Model file for the job. Use its own axes, mm. A direction names the side the tool comes from. Round coordinates to 2 decimals unless told otherwise and drop trailing zeros. Order: outer loops, then holes, each group sorted by start corner. A loop starts at its lowest first (then second) coordinate and runs counter-clockwise, first axis right, second up. Notation, with made-up numbers: M -33,76.5 L 14,76.5 A6 ccw 14,82.5 Z; hole C -9.75,-21.75 d6. An arc over 180 degrees is marked long. Return JSON: item names as keys, results as strings. Group by question number.
Item 1: Slice it at A-A on x = 105. Write the cut outline in (y, z), then the cut area to 3 significant figures.
Item 2: Which spindle directions (+Z, -Z, +X, -X, +Y, -Y) get a long thin tool onto all of the face, cutting with end or side? Do faces 5 (the face through (162, 117.5, 7)), 6 (the face through (180.505, 12.72, 198.768)), 7 (the face through (161.923, 28.755, 1.232)), 8 (the face through (14.479, 1.232, 188.966)). Say none if no direction does.
Item 3: Slice it at C-C on x = 15. Write the cut outline in (y, z), then the cut area to 3 significant figures.
Item 4: Slice it at B-B on y = 96. Write the cut outline in (x, z), then the cut area to 4 significant figures.
Item 5: Pin check, flat tips, straight feed: pin 1 Ø5 at (x, z) = (250.5, 37.5) entering from +Y; pin 2 Ø3 at (x, y) = (277.5, 115) entering from -Z. Stop position of each tip, or through.
Item 6: Probe line 1 along X through (y, z) = (25, 0.85); line 2 along Y through (x, z) = (195, 1.6); line 3 along X through (y, z) = (12, 145.5). List the from-to ranges inside material, lowest first.
Item 7: Slice it at D-D on z = 34. Write the cut outline in (x, y), then the cut area to 3 significant figures.
Item 8: Pull direction Y, two halves, no side cores. Call faces 1 (the face through (149, 120, 188)), 2 (the face through (148, 61, 0)), 3 (the face through (148.505, 12.72, 198.768)), 4 (the face through (148, 0, 99)): pulls with the +Y half, pulls with the -Y half, needs draft (parallel to the pull), parting line crosses it, or undercut.
from build123d import *

# Parameters (mm, degrees)
F0_W      = 300
F0_H      = 120
F1_DEPTH  = 200
F2_T      = -2.5
F3_W      = 297.5
F3_H      = 197.5
F3_W_2    = 277.5
F3_H_2    = 177.5
F4_DEPTH  = 2.5
F5_R      = 2
F6_DEPTH  = 200.001
F7_R      = 5
F8_DEPTH  = 5
F9_R      = 4
F10_DEPTH = 2.5
F11_R     = 12.5
F12_DEPTH = 3


with BuildPart() as f1:
    # F0 (on Top) → F1 (new body)
    with BuildSketch(Plane.XY):
        with Locations((150, 60)):
            Rectangle(F0_W, F0_H)
    extrude(amount=F1_DEPTH)

    # F2
    f2_openings = [f1.faces().sort_by_distance(p)[0] for p in [
        (150, 120, 100),
    ]]
    offset(amount=F2_T, openings=f2_openings)

    # F3 (on face) → F4 (join)
    with BuildSketch(Plane(origin=(0, 120, 0), x_dir=(-1, 0, 0), z_dir=(0, 1, 0))):
        with Locations((-148.75, 98.75)):
            Rectangle(F3_W, F3_H)
        with Locations((-148.75, 98.75)):
            Rectangle(F3_W_2, F3_H_2, mode=Mode.SUBTRACT)
    extrude(amount=-F4_DEPTH)

    # F5 (on face) → F6 (cut, through all)
    with BuildSketch(Plane.XY.offset(200)):
        with Locations((277.5, 115)):
            Circle(F5_R)
    extrude(amount=-F6_DEPTH, mode=Mode.SUBTRACT)

    # F7 (on face) → F8 (cut)
    with BuildSketch(Plane.XY.offset(200)):
        with Locations((185.5, 12.5)):
            Circle(F7_R)
        with Locations((153.5, 12.5)):
            Circle(F7_R)
        with Locations((121.5, 12.5)):
            Circle(F7_R)
        with Locations((89.5, 12.5)):
            Circle(F7_R)
        with Locations((57.5, 12.5)):
            Circle(F7_R)
        with Locations((25.5, 12.5)):
            Circle(F7_R)
    extrude(amount=-F8_DEPTH, mode=Mode.SUBTRACT)

    # F9 (on face) → F10 (cut)
    with BuildSketch(Plane.XZ):
        with Locations((285, 185)):
            Circle(F9_R)
        with Locations((285, 15)):
            Circle(F9_R)
        with Locations((15, 185)):
            Circle(F9_R)
        with Locations((15, 15)):
            Circle(F9_R)
    extrude(amount=-F10_DEPTH, mode=Mode.SUBTRACT)

    # F11 (on face) → F12 (cut)
    with BuildSketch(Plane.XY):
        with Locations((150, 25)):
            Circle(F11_R)
        with Locations((195, 25)):
            Circle(F11_R)
        with Locations((105, 25)):
            Circle(F11_R)
    extrude(amount=F12_DEPTH, mode=Mode.SUBTRACT)


solid = f1.part
Output values:
{
 "1": {"outline": "M 0,0 L 12.5,0 L 12.5,2.5 L 2.5,2.5 L 2.5,197.5 L 117.5,197.5 L 117.5,187.5 L 120,187.5 L 120,200 L 0,200 Z; M 37.5,0 L 120,0 L 120,10 L 117.5,10 L 117.5,2.5 L 37.5,2.5 Z", "area": "1,070 mm²"},
 "2": {"face 5": "none", "face 6": "+Z", "face 7": "-Z", "face 8": "-Y"},
 "3": {"outline": "M 0,0 L 120,0 L 120,10 L 117.5,10 L 117.5,2.5 L 2.5,2.5 L 2.5,11 L 0,11 Z; M 0,19 L 2.5,19 L 2.5,181 L 0,181 Z; M 0,189 L 2.5,189 L 2.5,197.5 L 117.5,197.5 L 117.5,187.5 L 120,187.5 L 120,200 L 0,200 Z", "area": "1,090 mm²"},
 "4": {"outline": "M 0,0 L 300,0 L 300,200 L 0,200 Z; hole M 2.5,2.5 L 297.5,2.5 L 297.5,197.5 L 2.5,197.5 Z", "area": "2,475 mm²"},
 "5": {"pin 1": "y = 2.5", "pin 2": "through"},
 "6": {"line 1": "0 to 92.5, 117.5 to 137.5, 162.5 to 182.5, 207.5 to 300", "line 2": "0 to 12.5, 37.5 to 120", "line 3": "0 to 2.5, 297.5 to 300"},
 "7": {"outline": "M 0,0 L 300,0 L 300,120 L 287.5,120 L 287.5,117.5 L 297.5,117.5 L 297.5,2.5 L 2.5,2.5 L 2.5,117.5 L 10,117.5 L 10,120 L 0,120 Z", "area": "1,380 mm²"},
 "8": {"face 1": "pulls with the +Y half", "face 2": "needs draft", "face 3": "undercut", "face 4": "pulls with the -Y half"}
}
